Read the model definition and answer for the solid it produces. Units are mm, in the model's axes. Face numbers are marked on the shaded views. A direction names the side the tool comes from. Coordinates: 2 decimals unless noted, no trailing zeros. Write each loop counter-clockwise with the first axis right and the second up, starting at its lowest first coordinate (ties: lowest second). Pieces come first, ordered by that corner, then holes. Notation, with made-up numbers: (33.25, 33.25) - (48.25, 33.25) arc R22 cw to (48.25, 41.25) - close; hole circle Ø8 at (18, 32). An arc over 180 degrees is marked (long way). Return JSON: item names as keys, results as strings.
```python
from build123d import *

# Parameters (mm, degrees)
F3_DEPTH = 63.5
F4_DEPTH = 25.4


with BuildPart() as f1:
    # F0 (on Top) → F1 (revolve)
    with BuildSketch(Plane.XY):
        with BuildLine():
            Line((-86.542711, 10.830558), (-86.542711, 6.004558))
            Line((-86.542711, 6.004558), (97.607289, 6.004558))
            Line((97.607289, 6.004558), (97.607289, 18.704558))
            Line((97.607289, 18.704558), (8.707289, 18.704558))
            ThreePointArc((8.707289, 18.704558), (4.54759, 14.187595), (-1.329683, 12.408912))
            ThreePointArc((-1.329683, 12.408912), (-1.624219, 12.40452), (-1.918771, 12.407566))
            Line((-1.918771, 12.407566), (-36.700717, 12.328112))
            ThreePointArc((-36.700717, 12.328112), (-38.280061, 13.575768), (-38.876261, 15.498142))
            Line((-38.876261, 15.498142), (-43.626061, 15.498142))
            ThreePointArc((-43.626061, 15.498142), (-45.254669, 13.356142), (-47.75214, 12.354558))
            ThreePointArc((-47.75214, 12.354558), (-48.315292, 12.323061), (-48.878444, 12.354558))
            Line((-48.878444, 12.354558), (-85.018711, 12.354558))
            ThreePointArc((-85.018711, 12.354558), (-86.096341, 11.908189), (-86.542711, 10.830558))
        make_face()
    revolve(axis=Axis((5.532289, 6.004558, 0), (1, 0, 0)))

    # F2 (on Front) → F3 (cut)
    with BuildSketch(Plane.XZ):
        with BuildLine():
            Line((-3.93209, 27.841151), (-3.93209, 6.35))
            ThreePointArc((-3.93209, 6.35), (10.307284, 2.745661), (24.945787, 1.535172))
            Line((24.945787, 1.535172), (95.049836, 1.535172))
            Line((95.049836, 1.535172), (97.884275, 0))
            Line((97.884275, 0), (100.466569, 1.535172))
            Line((100.466569, 1.535172), (113.435097, 10.608604))
            Line((113.435097, 10.608604), (113.435097, 27.841151))
            Line((113.435097, 27.841151), (97.66791, 27.841151))
            Line((97.66791, 27.841151), (-3.93209, 27.841151))
        make_face()
        with BuildLine():
            Line((100.466569, -1.535172), (97.884275, 0))
            Line((97.884275, 0), (95.049836, -1.535172))
            Line((95.049836, -1.535172), (24.945787, -1.535172))
            ThreePointArc((24.945787, -1.535172), (10.307284, -2.745661), (-3.93209, -6.35))
            Line((-3.93209, -6.35), (-3.93209, -27.841151))
            Line((-3.93209, -27.841151), (113.435097, -27.841151))
            Line((113.435097, -27.841151), (113.435097, -10.608604))
            Line((113.435097, -10.608604), (100.466569, -1.535172))
        make_face()
    extrude(amount=-F3_DEPTH, mode=Mode.SUBTRACT)

    # F2 (on Front) → F4 (cut)
    with BuildSketch(Plane.XZ):
        with BuildLine():
            Line((-3.93209, 27.841151), (-3.93209, 6.35))
            ThreePointArc((-3.93209, 6.35), (10.307284, 2.745661), (24.945787, 1.535172))
            Line((24.945787, 1.535172), (95.049836, 1.535172))
            Line((95.049836, 1.535172), (97.884275, 0))
            Line((97.884275, 0), (100.466569, 1.535172))
            Line((100.466569, 1.535172), (113.435097, 10.608604))
            Line((113.435097, 10.608604), (113.435097, 27.841151))
            Line((113.435097, 27.841151), (97.66791, 27.841151))
            Line((97.66791, 27.841151), (-3.93209, 27.841151))
        make_face()
        with BuildLine():
            Line((100.466569, -1.535172), (97.884275, 0))
            Line((97.884275, 0), (95.049836, -1.535172))
            Line((95.049836, -1.535172), (24.945787, -1.535172))
            ThreePointArc((24.945787, -1.535172), (10.307284, -2.745661), (-3.93209, -6.35))
            Line((-3.93209, -6.35), (-3.93209, -27.841151))
            Line((-3.93209, -27.841151), (113.435097, -27.841151))
            Line((113.435097, -27.841151), (113.435097, -10.608604))
            Line((113.435097, -10.608604), (100.466569, -1.535172))
        make_face()
    extrude(amount=F4_DEPTH, mode=Mode.SUBTRACT)


solid = f1.part
```
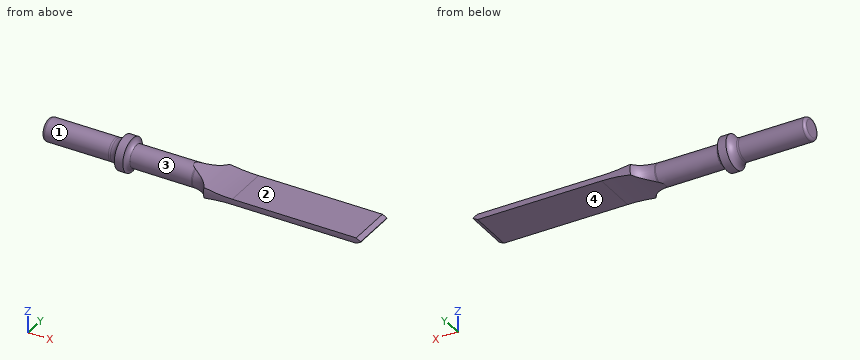
(1) Determine the mould class of the marked faces 3 and 4 for opening direction X: +X half, -X half, draft (parallel to the pull), parting line (faces both ways), or undercut.
Answer:
{"face 3": "undercut", "face 4": "draft"}
(2) A cutting plane is placed at A-A (x = 49.5). Determine the outline of the cut face in (y, z), and give its area (3 significant figures).
Answer:
{"outline": "(-6.6, -1.54) - (18.61, -1.54) arc R12.7 ccw to (18.61, 1.54) - (-6.6, 1.54) arc R12.7 ccw to start", "area": "77.8 mm²"}
(3) Straight lines are drawn through the part: line 1 (Z direction, x = 55.5, y = 12.75); line 2 (Y direction, x = -63, z = 0.25); line 3 (Z direction, x = -16, y = 5.75). For each, find the intervals that lie inside material, in ascending order. Write a range as from..to.
Answer:
{"line 1": "-1.54..1.54", "line 2": "-0.34..12.35", "line 3": "-6.37..6.37"}
(4) A cutting plane is placed at B-B (x = -34). Determine the outline of the cut face in (y, z).
Answer:
{"outline": "circle Ø12.66 at (6, 0)"}
(5) Which of the six approach directions +Z, -Z, +X, -X, +Y, -Y give full straight-line access (tool end or side, diameter ignored) to the marked faces 1 and 2?
Answer:
{"face 1": "-X", "face 2": "+Z, +X, +Y, -Y"}
(6) Flat-ended cylindrical pins translate along their axes: P1, Ø7.5, axis at x = 44, y = 11.5, coming from the -Z side; P2, Ø3, axis at x = 36, y = 3, coming from the +Z side. Find the tip coordinate at first contact, or state that the pin passes through.
Answer:
{"P1": "z = -1.54", "P2": "z = 1.54"}
